The model under review builds one solid part; all positions refer to its coordinate system, in mm. Round coordinates to 2 decimals unless told otherwise and drop trailing zeros. Loops run counter-clockwise (first coordinate to the right, second up) from the corner with the lowest first, then second, coordinate; pieces in that order, holes last. Notation, with made-up numbers: M -33.75,70 L -13.75,70 A8 ccw -13.75,77 Z; hole C 56,84 d8. An arc over 180 degrees is marked long. Answer in a Markdown table with one row per item. Add a question column.
from build123d import *

# Parameters (mm, degrees)
SKETCH_1_R               = 50
EXTRUDE_1_DEPTH          = 12
SKETCH_4_R               = 5.075
CUT_EXTRUDE_5_DEPTH      = 72.721684308
PATTERN_CIRCULAR_3_COUNT = 6
SKETCH_27_R              = 42
CUT_EXTRUDE_7_DEPTH      = 72.721684464


with BuildPart() as part:
    # 草图1 → 凸台-拉伸1 (new body)
    with BuildSketch(Plane(origin=(0, 0, 0), x_dir=(1, 0, 0), z_dir=(0, 1, 0))):
        with Locations(Location((0, 0, 0), (0, 0, 270))):
            Circle(SKETCH_1_R)
    extrude(amount=EXTRUDE_1_DEPTH)

    # 草图4 → 切除-拉伸5 (cut, through all)
    with BuildSketch(Plane.XY):
        with Locations((0, 6.19163712)):
            Circle(SKETCH_4_R)
    cut_extrude_5 = extrude(amount=-CUT_EXTRUDE_5_DEPTH, mode=Mode.SUBTRACT)

    # 阵列(圆周)3: 切除-拉伸5 ×6 about axis
    pattern_circular_3_axis = Axis((0, 0, 0), (0, 1, 0))
    for i in range(1, PATTERN_CIRCULAR_3_COUNT):
        add(cut_extrude_5.rotate(pattern_circular_3_axis, i * 360 / PATTERN_CIRCULAR_3_COUNT), mode=Mode.SUBTRACT)

    # 草图27 → 切除-拉伸7 (cut, through all)
    with BuildSketch(Plane.XZ):
        with Locations(Location((0, 0, 0), (0, 0, 270))):
            Circle(SKETCH_27_R)
    extrude(amount=-CUT_EXTRUDE_7_DEPTH, mode=Mode.SUBTRACT)


solid = part.part
1. Take a section at C-C, the plane y = 9.75. State the section outline as (x, z) points, and give its area (3 significant figures).
2. Take a section at B-B, the plane x = 0. State the section outline as (y, z) points.
3. Take a section at D-D, the plane x = -30. State the section outline as (y, z) points, and give its area (3 significant figures).
4. Mouldability with a two-part tool opening along Z and no side actions: class faces 1 (the flat face through (41, 0, -11)), 2 (the cylindrical face through (15.02, 5.92, 47.69)), 3 (the cylindrical face through (-39.984, 11.223, -22.322)) as released by +Z, released by -Z, zero draft, split by the parting line, or undercut.
5. For pin 1 Ø1 at (y, z) = (10.5, 5.5) entering from +X; pin 2 Ø8 at (x, z) = (-39, -12) entering from +Y; pin 3 Ø3 at (x, y) = (32.5, 8) entering from +Z; pin 4 Ø5 at (y, z) = (8, -33) entering from -X, all flat-tipped, find the tip position at first contact; note any pin that passes through.
6. Take a section at A-A, the plane z = 0. State the section outline as (x, y) points.
7. To check wall thickness, follow probe 1 along Y at (x, z) = (0, 47.75); probe 2 along X at (y, z) = (5, 0); probe 3 along X at (y, z) = (9, 11) (3 decimals). State the ranges of each line that lie inside material, in increasing order.
Check sheet entries:
| question | item | result |
|---|---|---|
| 1 | outline | M -45,-21.8 L -38.05,-17.79 A42 cw -38.05,17.79 L -45,21.8 A50 ccw Z; M -41.38,-28.07 A50 ccw -3.62,-49.87 L -3.62,-41.84 A42 cw -34.43,-24.06 Z; M -41.38,28.07 L -34.43,24.06 A42 cw -3.62,41.84 L -3.62,49.87 A50 ccw Z; M 3.62,-49.87 A50 ccw 41.38,-28.07 L 34.43,-24.06 A42 cw 3.62,-41.84 Z; M 3.62,41.84 A42 cw 34.43,24.06 L 41.38,28.07 A50 ccw 3.62,49.87 Z; M 38.05,-17.79 L 45,-21.8 A50 ccw 45,21.8 L 38.05,17.79 A42 cw Z |
| 1 | area | 1,960 mm^2 |
| 2 | outline | M 0,-50 L 1.12,-50 L 1.12,-42 L 0,-42 Z; M 0,42 L 1.12,42 L 1.12,50 L 0,50 Z; M 11.27,-50 L 12,-50 L 12,-42 L 11.27,-42 Z; M 11.27,42 L 12,42 L 12,50 L 11.27,50 Z |
| 3 | outline | M 0,-40 L 12,-40 L 12,-29.39 L 0,-29.39 Z; M 0,29.39 L 12,29.39 L 12,40 L 0,40 Z |
| 3 | area | 255 mm^2 |
| 4 | face 1 | zero draft |
| 4 | face 2 | split by the parting line |
| 4 | face 3 | undercut |
| 5 | pin 1 | stops at x = 49.75 |
| 5 | pin 2 | stops at y = 12 |
| 5 | pin 3 | stops at z = 39.23 |
| 5 | pin 4 | stops at x = -39.62 |
| 6 | outline | M -50,0 L -42,0 L -42,12 L -50,12 Z; M 42,0 L 50,0 L 50,12 L 42,12 Z |
| 7 | probe 1 | y = 0 to 1.12, 11.27 to 12 |
| 7 | probe 2 | x = -50 to -42, 42 to 50 |
| 7 | probe 3 | x = -48.775 to -40.534, 40.534 to 48.775 |
